Geometry check sheet. Reference: the model listing, model coordinates, mm. A direction names the side the tool comes from. Coordinates: 2 decimals unless noted, no trailing zeros. Write each loop counter-clockwise with the first axis right and the second up, starting at its lowest first coordinate (ties: lowest second). Pieces come first, ordered by that corner, then holes.
from build123d import *

# Parameters (mm, degrees)
BOSS_EXTRUDE1_DEPTH = 35
SKETCH9_R           = 5
BOSS_EXTRUDE3_DEPTH = 13
SKETCH10_W          = 39.744762059
SKETCH10_H          = 6.949903748
CUT_EXTRUDE1_DEPTH  = 13
SKETCH12_R          = 3
CUT_EXTRUDE3_DEPTH  = 51.56128384


with BuildPart() as part:
    # Sketch4 → Boss-Extrude1 (new, symmetric)
    with BuildSketch(Plane.XY):
        with BuildLine():
            Line((7.5, -2.9), (-7.5, -2.9))
            ThreePointArc((-7.5, -2.9), (-10.4, 0), (-7.5, 2.9))
            Line((-7.5, 2.9), (7.5, 2.9))
            ThreePointArc((7.5, 2.9), (10.4, 0), (7.5, -2.9))
        make_face()
        with BuildLine():
            Line((7.5, -1.9), (-7.5, -1.9))
            ThreePointArc((-7.5, -1.9), (-9.4, 0), (-7.5, 1.9))
            Line((-7.5, 1.9), (7.5, 1.9))
            ThreePointArc((7.5, 1.9), (9.4, 0), (7.5, -1.9))
        make_face(mode=Mode.SUBTRACT)
    extrude(amount=BOSS_EXTRUDE1_DEPTH, both=True)

    # Sketch9 → Boss-Extrude3 (add, symmetric)
    with BuildSketch(Plane(origin=(0, 0, 0), x_dir=(0, 0, -1), z_dir=(1, 0, 0))):
        with Locations((-39.073082371, 0.015275052)):
            Circle(SKETCH9_R)
    extrude(amount=BOSS_EXTRUDE3_DEPTH, both=True)

    # Sketch10 → Cut-Extrude1 (cut, symmetric)
    with BuildSketch(Plane(origin=(0, 0, 0), x_dir=(1, 0, 0), z_dir=(0, 1, 0))):
        with Locations((-2.189570447, -46.548034245)):
            Rectangle(SKETCH10_W, SKETCH10_H)
    extrude(amount=CUT_EXTRUDE1_DEPTH, both=True, mode=Mode.SUBTRACT)

    # Sketch12 → Cut-Extrude3 (cut, through all)
    with BuildSketch(Plane(origin=(13, 0, 0), x_dir=(0, 0, -1), z_dir=(1, 0, 0))):
        with Locations((-39.073082371, 0.015275052)):
            Circle(SKETCH12_R)
    extrude(amount=-CUT_EXTRUDE3_DEPTH, mode=Mode.SUBTRACT)


solid = part.part
1. Thickness scan on line 1 along X through (y, z) = (0.25, -29.5); line 2 along Y through (x, z) = (-7.75, 28); line 3 along Y through (x, z) = (10.25, 39). Record the ranges inside material, lowest first.
Computed values:
line 1: x = -10.39 to -9.38, 9.38 to 10.39
line 2: y = -2.89 to -1.88, 1.88 to 2.89
line 3: y = -4.98 to -2.98, 3.01 to 5.01
2. Sectioned sample at A-A, the plane z = -18. Record the boundary of the cut face in (x, y), and give its area (3 significant figures).
Computed values:
outline: (-7.5, -2.9) - (7.5, -2.9) arc R2.9 ccw to (7.5, 2.9) - (-7.5, 2.9) arc R2.9 ccw to start; hole (-7.5, -1.9) - (7.5, -1.9) arc R1.9 ccw to (7.5, 1.9) - (-7.5, 1.9) arc R1.9 ccw to start
area: 45.1 mm2
3. Draft check along Y on faces 5 (the flat face through (0, -2.9, 0)), 6 (the cylindrical face through (0.132, -0.029, 34.073)), 7 (the cylindrical face through (-10.4, -0.1, 0.5)), 8 (the flat face through (13, 2.3, 36.6)). Enter one of: released by +Y, released by -Y, zero draft, split by the parting line, or undercut.
Computed values:
face 5: released by -Y
face 6: undercut
face 7: split by the parting line
face 8: zero draft
4. Gauge pin test, flat ends, axial feed: pin 1 Ø6 at (x, y) = (-7, -3.5) entering from +Z; pin 2 Ø4.5 at (x, z) = (-1, -17) entering from +Y; pin 3 Ø2 at (y, z) = (3, -15) entering from +X; pin 4 Ø12 at (x, z) = (-3, -0.5) entering from -Y. Record the tip position at first contact, or that the pin passes through.
Computed values:
pin 1: stops at z = 43.07
pin 2: stops at y = 2.9
pin 3: stops at x = 9.6
pin 4: stops at y = -2.9
5. Access from +Z, -Z, +X, -X, +Y, -Y to the whole of each face (thin tool, end or side, straight path). Record for faces 1 (the flat face through (0, 2.9, 0)), 2 (the cylindrical face through (-9.4, 0, 0.2)), 3 (the flat face through (0, 0, 43.073)), 4 (the cylindrical face through (10.4, 0.1, 0.5)).
Computed values:
face 1: -Z, +X, -X, +Y
face 2: -Z
face 3: +Z, +X, -X, +Y, -Y
face 4: -Z, +X
